Print and shaded views of the part. All mm, measured from the part's lowest x, y and z. A direction names the side the tool comes from. Round coordinates to 2 decimals unless told otherwise and drop trailing zeros. Loops run counter-clockwise (first coordinate to the right, second up) from the corner with the lowest first, then second, coordinate; pieces in that order, holes last. Notation, with made-up numbers: (29, 74) - (58, 74) arc R19 ccw to (58, 105) - close; hole circle Ø9 at (75.25, 4.5). An arc over 180 degrees is marked (long way). Answer as a JSON object with one key per item and string values.
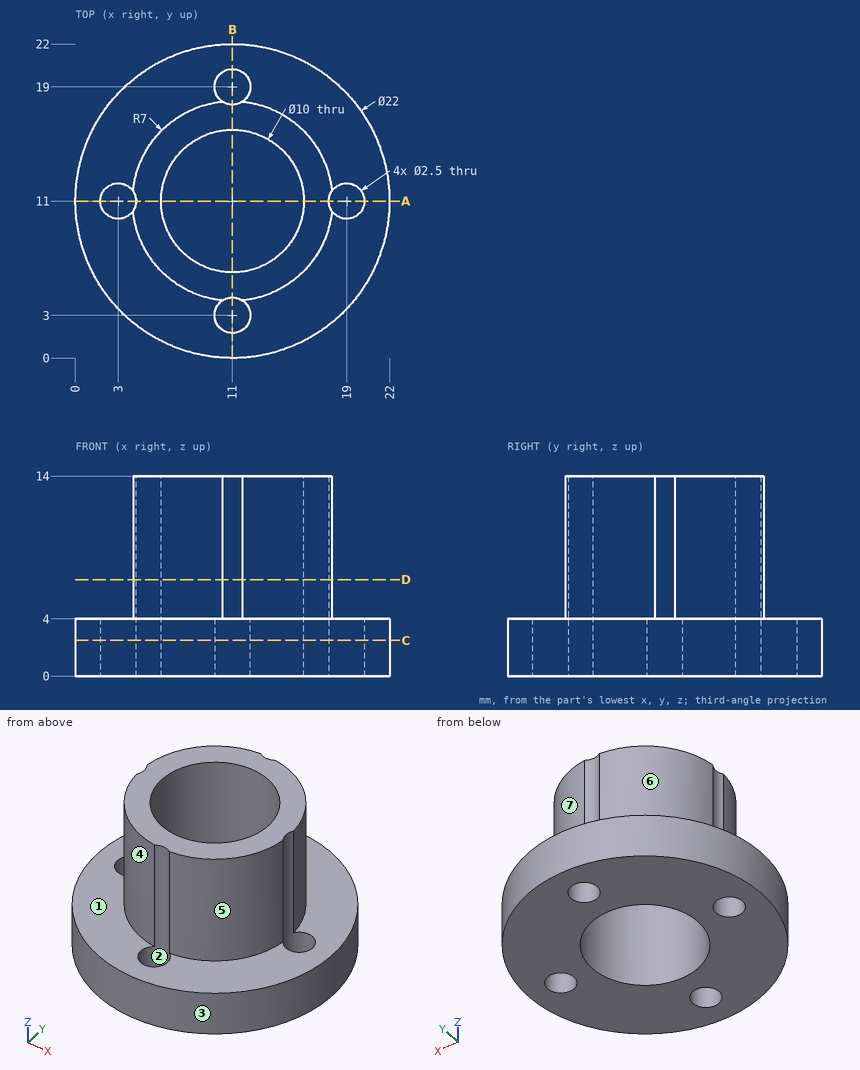
1) Drop flat-ended pins along their axis: P1, Ø1, axis at y = 16.5, z = 3.5, coming from the -X side; P2, Ø4, axis at y = 6, z = 5, coming from the -X side; P3, Ø3, axis at y = 5.5, z = 3, coming from the +X side; P4, Ø2, axis at x = 11, y = 19, coming from the +Z side. Give the stop position or say it passes through.
Values follow:
{"P1": "x = 1.2", "P2": "x = 0.5", "P3": "x = 21.25", "P4": "through"}
2) Two-plate mould, pull along X, no slides. Class the marked faces 1, 2 and 3: pulls with the +X half, pulls with the -X half, needs draft (parallel to the pull), parting line crosses it, or undercut.
Values follow:
{"face 1": "needs draft", "face 2": "undercut", "face 3": "parting line crosses it"}
3) Probe probe 1 along Y at (x, z) = (10.25, 1.25); probe 2 along Z at (x, y) = (5, 7.25); probe 3 along X at (y, z) = (12.75, 8.25). List the from-to ranges inside material, lowest first.
Values follow:
{"probe 1": "0.03 to 2, 4 to 6.06, 15.94 to 18, 20 to 21.97", "probe 2": "0 to 4", "probe 3": "4.22 to 6.32, 15.68 to 17.78"}
4) Tool access for the marked faces 4, 5, 6 and 7: list every direction of +Z, -Z, +X, -X, +Y, -Y with a clear straight run to the whole face (end or side of a thin tool).
Values follow:
{"face 4": "+Z, -X, -Y", "face 5": "+Z, +X, -Y", "face 6": "+Z, -X, +Y", "face 7": "+Z, +X, +Y"}
5) Slice it at A-A on y = 11. List the corners of the cut face in (x, z), then the cut area to 3 significant figures.
Values follow:
{"outline": "(0, 0) - (1.75, 0) - (1.75, 4) - (0, 4) - close; (4.25, 0) - (6, 0) - (6, 14) - (4.25, 14) - close; (16, 0) - (17.75, 0) - (17.75, 14) - (16, 14) - close; (20.25, 0) - (22, 0) - (22, 4) - (20.25, 4) - close", "area": "63.0 mm²"}
6) Slice it at D-D on z = 6.75. List the corners of the cut face in (x, y).
Values follow:
{"outline": "(4.04, 10.3) arc R7 ccw to (10.3, 4.04) arc R1.25 cw to (11.7, 4.04) arc R7 ccw to (17.96, 10.3) arc R1.25 cw to (17.96, 11.7) arc R7 ccw to (11.7, 17.96) arc R1.25 cw to (10.3, 17.96) arc R7 ccw to (4.04, 11.7) arc R1.25 cw to start; hole circle Ø10 at (11, 11)"}
7) Slice it at C-C on z = 2.5. List the corners of the cut face in (x, y).
Values follow:
{"outline": "circle Ø22 at (11, 11); hole circle Ø2.5 at (3, 11); hole circle Ø10 at (11, 11); hole circle Ø2.5 at (11, 3); hole circle Ø2.5 at (11, 19); hole circle Ø2.5 at (19, 11)"}
